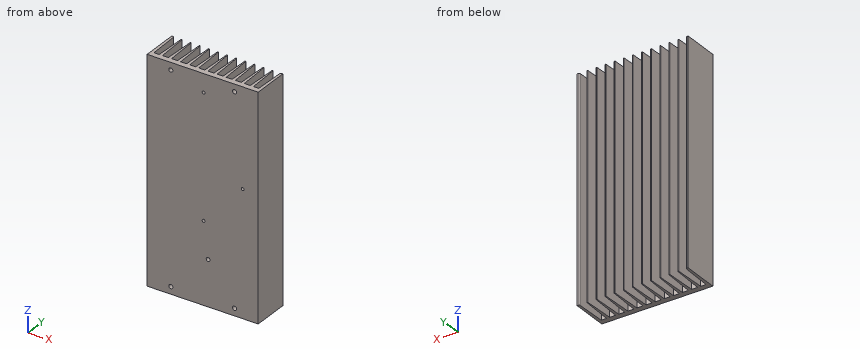
from build123d import *

# Parameters (mm, degrees)
EXTRUDE_1_DEPTH       = 244
EXTRUDE_3_DEPTH       = 244
PATTERN_CURVE_1_DEPTH = 244
SKETCH_3_R            = 2.25
CUT_EXTRUDE_1_DEPTH   = 6
SKETCH_4_R            = 2.1
SKETCH_4_R_2          = 1.6
CUT_EXTRUDE_2_DEPTH   = 6


# Read off the part's stored shape, not the designer's step: the pattern curve step
with BuildPart() as part:
    # Sketch 1 → Extrude 1 (new body)
    with BuildSketch(Plane.XY):
        with BuildLine():
            Line((0, 40), (1.528979332, 40))
            ThreePointArc((1.528979332, 40), (2.225614441, 39.717425624), (2.528547087, 39.029399052))
            Line((2.528547087, 39.029399052), (3.5, 6))
            Line((3.5, 6), (118.5, 6))
            Line((118.5, 6), (119.471452913, 39.029399052))
            ThreePointArc((119.471452913, 39.029399052), (119.774385559, 39.717425624), (120.471020668, 40))
            Line((120.471020668, 40), (122, 40))
            Line((122, 40), (122, 0))
            Line((122, 0), (0, 0))
            Line((0, 0), (0, 40))
        make_face()
    extrude(amount=EXTRUDE_1_DEPTH)

    # Sketch 2 → Extrude 3 (add)
    with BuildSketch(Plane.XY.offset(244)):
        with BuildLine():
            Line((10.5, 39.5), (9.25, 6))
            Line((9.25, 6), (12.75, 6))
            Line((12.75, 6), (11.5, 39.5))
            ThreePointArc((11.5, 39.5), (11, 40), (10.5, 39.5))
        make_face()
    extrude(amount=-EXTRUDE_3_DEPTH)

    # Pattern Curve 1 outline → Pattern Curve 1 (add)
    with BuildSketch(Plane.XY):
        with BuildLine():
            ThreePointArc((21.5, 39.5), (21, 40), (20.5, 39.5))
            Line((20.5, 39.5), (19.25, 6))
            Line((19.25, 6), (22.75, 6))
            Line((22.75, 6), (21.5, 39.5))
        make_face()
        with BuildLine():
            Line((110.5, 39.5), (109.25, 6))
            Line((109.25, 6), (112.75, 6))
            Line((112.75, 6), (111.5, 39.5))
            ThreePointArc((111.5, 39.5), (111, 40), (110.5, 39.5))
        make_face()
        with BuildLine():
            Line((100.5, 39.5), (99.25, 6))
            Line((99.25, 6), (102.75, 6))
            Line((102.75, 6), (101.5, 39.5))
            ThreePointArc((101.5, 39.5), (101, 40), (100.5, 39.5))
        make_face()
        with BuildLine():
            Line((90.5, 39.5), (89.25, 6))
            Line((89.25, 6), (92.75, 6))
            Line((92.75, 6), (91.5, 39.5))
            ThreePointArc((91.5, 39.5), (91, 40), (90.5, 39.5))
        make_face()
        with BuildLine():
            Line((80.5, 39.5), (79.25, 6))
            Line((79.25, 6), (82.75, 6))
            Line((82.75, 6), (81.5, 39.5))
            ThreePointArc((81.5, 39.5), (81, 40), (80.5, 39.5))
        make_face()
        with BuildLine():
            Line((70.5, 39.5), (69.25, 6))
            Line((69.25, 6), (72.75, 6))
            Line((72.75, 6), (71.5, 39.5))
            ThreePointArc((71.5, 39.5), (71, 40), (70.5, 39.5))
        make_face()
        with BuildLine():
            Line((60.5, 39.5), (59.25, 6))
            Line((59.25, 6), (62.75, 6))
            Line((62.75, 6), (61.5, 39.5))
            ThreePointArc((61.5, 39.5), (61, 40), (60.5, 39.5))
        make_face()
        with BuildLine():
            Line((50.5, 39.5), (49.25, 6))
            Line((49.25, 6), (52.75, 6))
            Line((52.75, 6), (51.5, 39.5))
            ThreePointArc((51.5, 39.5), (51, 40), (50.5, 39.5))
        make_face()
        with BuildLine():
            Line((40.5, 39.5), (39.25, 6))
            Line((39.25, 6), (42.75, 6))
            Line((42.75, 6), (41.5, 39.5))
            ThreePointArc((41.5, 39.5), (41, 40), (40.5, 39.5))
        make_face()
        with BuildLine():
            Line((30.5, 39.5), (29.25, 6))
            Line((29.25, 6), (32.75, 6))
            Line((32.75, 6), (31.5, 39.5))
            ThreePointArc((31.5, 39.5), (31, 40), (30.5, 39.5))
        make_face()
    extrude(amount=PATTERN_CURVE_1_DEPTH)

    # Sketch 3 → Cut-Extrude 1 (cut)
    with BuildSketch(Plane.XZ):
        with Locations((26, 236)):
            Circle(SKETCH_3_R)
        with Locations((96, 236)):
            Circle(SKETCH_3_R)
        with Locations(Location((96, 8, 0), (0, 0, 180))):
            Circle(SKETCH_3_R)
        with Locations(Location((26, 8, 0), (0, 0, 180))):
            Circle(SKETCH_3_R)
    extrude(amount=-CUT_EXTRUDE_1_DEPTH, mode=Mode.SUBTRACT)

    # Sketch 4 → Cut-Extrude 2 (cut)
    with BuildSketch(Plane(origin=(1.487985642, 0, 27.400529356), x_dir=(1, 0, 0), z_dir=(0, -1, 0))):
        with Locations((65.512014358, 22.599470644)):
            Circle(SKETCH_4_R)
        with Locations((103.512014358, 109.099470644)):
            Circle(SKETCH_4_R_2)
        with Locations((60.512014358, 196.599470644)):
            Circle(SKETCH_4_R_2)
        with Locations((60.512014358, 61.599470644)):
            Circle(SKETCH_4_R_2)
    extrude(amount=-CUT_EXTRUDE_2_DEPTH, mode=Mode.SUBTRACT)


solid = part.part
Could you check a few things on this model? Use its own coordinates, in mm. Give positions to 0.01 mm unless a question says otherwise; leave off trailing zeros. Order: outer loops, then holes, each group sorted by start corner. A loop starts at its lowest first (then second) coordinate and runs counter-clockwise, first axis right, second up. Notation, with made-up numbers: (27, 58) -> (49, 58) arc R33 cw to (49, 94) -> close; hole circle Ø9 at (76, 48). An arc over 180 degrees is marked (long way). Return JSON: item names as keys, results as strings.
1. Imagine slicing it at A-A on z = 236. Give the number of separate pieces and of enclosed holes in the cut face, then the cut area to 3 significant figures.
Answer list:
{"separate pieces": "3", "enclosed holes": "0", "area": "1,720 mm2"}
2. I need wall thicknesses on line 1 (Z direction, x = 96, y = 4.65); line 2 (Z direction, x = 67, y = 2.65); line 3 (X direction, y = 3.25, z = 89). Which ranges of each line are inside material? Lowest first, please. Write a range as from..to.
Answer list:
{"line 1": "z = 0..5.75, 10.25..233.75, 238.25..244", "line 2": "z = 0..47.9, 52.1..244", "line 3": "x = 0..60.4, 63.6..122"}
3. For pin 1 Ø3 at (x, z) = (107, 78.5) entering from +Y; pin 2 Ø2.5 at (x, z) = (96, 236) entering from -Y; pin 3 Ø1.9 at (x, z) = (62, 89) entering from +Y, each with a flat end and sliding along its axis, tell me the tip position at first contact or that it passes through.
Answer list:
{"pin 1": "stops at y = 6", "pin 2": "passes through", "pin 3": "stops at y = 40"}
4. Imagine slicing it at B-B on x = 35.5. List the corners of the cut face in (y, z) for me, then the cut area to 3 significant figures.
Answer list:
{"outline": "(0, 0) -> (6, 0) -> (6, 244) -> (0, 244) -> close", "area": "1,460 mm2"}
